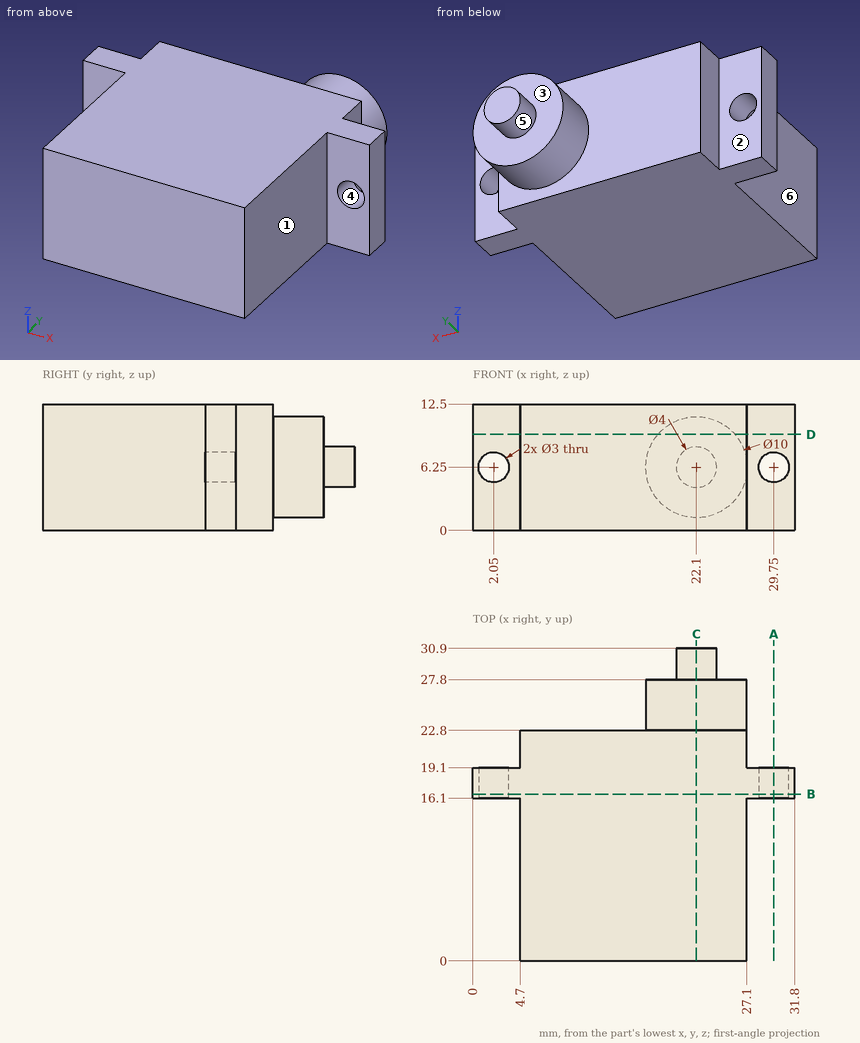
Drawing for the job (mm, zero at the part's lowest x, y, z). A direction names the side the tool comes from. Give positions to 0.01 mm unless a question says otherwise; leave off trailing zeros. Loops run counter-clockwise (first coordinate to the right, second up) from the corner with the lowest first, then second, coordinate; pieces in that order, holes last. Notation, with made-up numbers: (8.5, 73) - (50.5, 73) arc R11 ccw to (50.5, 91) - close; hole circle Ø11 at (-25, 86). An arc over 180 degrees is marked (long way). Write item = value, one per line. Start each with the question number.
1) Tool access for the marked faces 1, 2 and 3: list every direction of +Z, -Z, +X, -X, +Y, -Y with a clear straight run to the whole face (end or side of a thin tool).
2) Probe probe 1 along X at (y, z) = (18.45, 6.25); probe 2 along Z at (x, y) = (29.75, 16.95); probe 3 along Y at (x, z) = (9, 5.75). List the from-to ranges inside material, lowest first. Write a range as from..to.
3) Band-saw the part on B-B on y = 16.5. Give the cut face in (x, z), plus the area to 3 significant figures.
4) Band-saw the part on A-A on x = 29.75. Give the cut face in (y, z).
5) Drop flat-ended pins along their axis: pin 1 Ø2.5 at (x, z) = (1, 8) entering from -Y; pin 2 Ø4 at (x, z) = (1.5, 7) entering from +Y; pin 3 Ø1.5 at (y, z) = (11, 5) entering from +X. Give the stop position or say it passes through.
6) Pull direction Z, two halves, no side cores. Call the marked faces 4, 5 and 6: +Z half, -Z half, draft (parallel to the pull), parting line (faces both ways), or undercut.
7) Band-saw the part on D-D on z = 9.5. Give the cut face in (x, y).
8) Band-saw the part on C-C on x = 22.1. Give the cut face in (y, z), plus the area to 3 significant figures.
Final values:
q1.face_1 = +Z, -Z, +X, -Y
q1.face_2 = +Z, -Z, -X, +Y
q1.face_3 = +Y
q2.probe_1 = 0..0.55, 3.55..28.25, 31.25..31.8
q2.probe_2 = 0..4.75, 7.75..12.5
q2.probe_3 = 0..22.8
q3.outline = (0, 0) - (31.8, 0) - (31.8, 12.5) - (0, 12.5) - close; hole circle Ø3 at (2.05, 6.25); hole circle Ø3 at (29.75, 6.25)
q3.area = 383 mm²
q4.outline = (16.1, 0) - (19.1, 0) - (19.1, 4.75) - (16.1, 4.75) - close; (16.1, 7.75) - (19.1, 7.75) - (19.1, 12.5) - (16.1, 12.5) - close
q5.pin_1 = 16.1
q5.pin_2 = 19.1
q5.pin_3 = 27.1
q6.face_4 = undercut
q6.face_5 = parting line
q6.face_6 = draft
q7.outline = (0, 16.1) - (4.7, 16.1) - (4.7, 0) - (27.1, 0) - (27.1, 16.1) - (31.8, 16.1) - (31.8, 19.1) - (27.1, 19.1) - (27.1, 22.8) - (25.9, 22.8) - (25.9, 27.8) - (18.3, 27.8) - (18.3, 22.8) - (4.7, 22.8) - (4.7, 19.1) - (0, 19.1) - close
q8.outline = (0, 0) - (22.8, 0) - (22.8, 1.25) - (27.8, 1.25) - (27.8, 4.25) - (30.9, 4.25) - (30.9, 8.25) - (27.8, 8.25) - (27.8, 11.25) - (22.8, 11.25) - (22.8, 12.5) - (0, 12.5) - close
q8.area = 347 mm²
